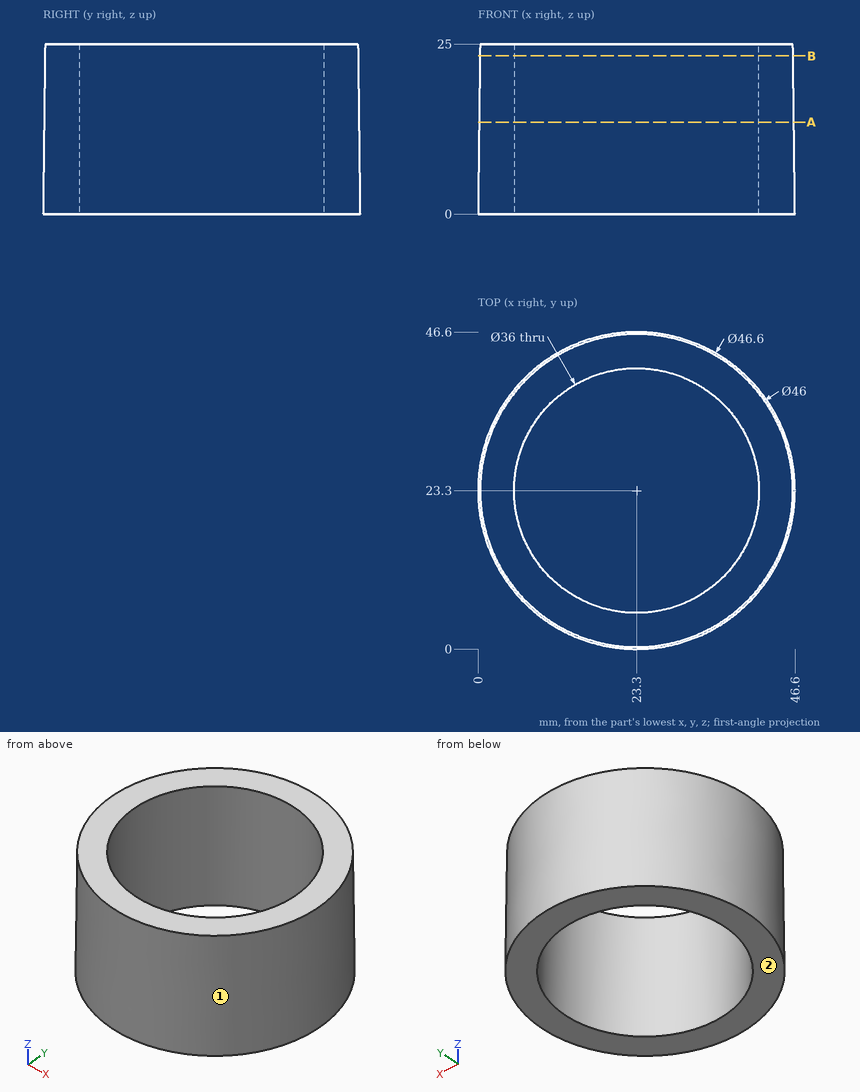
The figure shows three views and two pictorial views of one solid part (mm, origin at its lowest corner). Answer the questions. A direction names the side the tool comes from. Coordinates: 2 decimals unless noted, no trailing zeros. Write each loop counter-clockwise with the first axis right and the second up, starting at its lowest first coordinate (ties: lowest second). Pieces come first, ordered by that corner, then holes. Notation, with made-up numbers: (16.5, 59) -> (62.5, 59) arc R27 ccw to (62.5, 82) -> close; hole circle Ø8 at (88.5, -9). An arc over 180 degrees is marked (long way). Return JSON: item names as keys, results as strings.
1. A cutting plane is placed at B-B (z = 23.25). Determine the outline of the cut face in (x, y).
Found:
{"outline": "circle Ø46.04 at (23.3, 23.3); hole circle Ø36 at (23.3, 23.3)"}
2. Find the intervals of material crossed by line 1 along Y through (x, z) = (18.5, 12.25); line 2 along X through (y, z) = (23.3, 7); line 3 along X through (y, z) = (36.5, 15), in increasing order. Write a range as from..to.
Found:
{"line 1": "0.65..5.95, 40.65..45.95", "line 2": "0.08..5.3, 41.3..46.52", "line 3": "4.32..11.06, 35.54..42.28"}
3. Each of these flat-tipped pins is pushed along its axis until it touches: P1, Ø8, axis at x = 40, z = 19.5, coming from the -Y side; P2, Ø8, axis at y = 27.5, z = 17, coming from the -X side; P3, Ø2, axis at x = 12.5, z = 12.5, coming from the -Y side. Where does it stop, or does it pass through?
Found:
{"P1": "y = 4.04", "P2": "x = 0.19", "P3": "y = 2.33"}
4. A cutting plane is placed at A-A (z = 13.5). Determine the outline of the cut face in (x, y), and give its area (3 significant figures).
Found:
{"outline": "circle Ø46.28 at (23.3, 23.3); hole circle Ø36 at (23.3, 23.3)", "area": "664 mm2"}
5. A tool of negligible diameter and unlimited length cuts with its end or side. For the marked faces 1 and 2, from which of +Z, -Z, +X, -X, +Y, -Y can it reach the whole face along a straight path? Write none if from no direction.
Found:
{"face 1": "+Z", "face 2": "-Z, +X, -X, +Y, -Y"}
